CAD build for the part. Positions are in the model's coordinates, mm. Face numbers are marked on the shaded views. A direction names the side the tool comes from. Give positions to 0.01 mm unless a question says otherwise; leave off trailing zeros. Loops run counter-clockwise (first coordinate to the right, second up) from the corner with the lowest first, then second, coordinate; pieces in that order, holes last. Notation, with made-up numbers: M 53,-18 L 92,-18 A22 ccw 92,12 Z; hole C 14.5,-35.75 d3. An arc over 180 degrees is marked long. One line per question, with ' | ' between items.
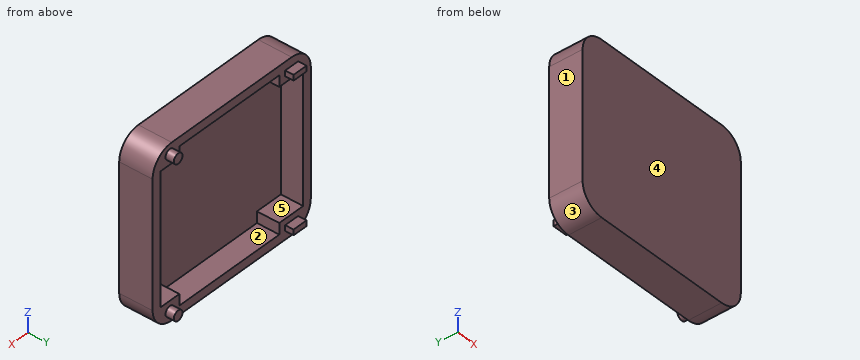
```python
from build123d import *

# Parameters (mm, degrees)
SKETCH1_W           = 84.074
SKETCH1_H           = 77.724
BOSS_EXTRUDE1_DEPTH = 5.08
SKETCH2_W           = 84.074
SKETCH2_H           = 77.724
BOSS_EXTRUDE2_DEPTH = 10.16
FILLET1_R           = 10.16
SKETCH3_R           = 2.286
SKETCH3_W           = 6.858
SKETCH3_H           = 2.54
BOSS_EXTRUDE3_DEPTH = 3.81


with BuildPart() as part:
    # Sketch1 → Boss-Extrude1 (new body)
    with BuildSketch(Plane(origin=(0, 0, 0), x_dir=(1, 0, 0), z_dir=(0, 1, 0))):
        Rectangle(SKETCH1_W, SKETCH1_H)
    extrude(amount=BOSS_EXTRUDE1_DEPTH)

    # Sketch2 → Boss-Extrude2 (add)
    with BuildSketch(Plane(origin=(0, 5.08, 0), x_dir=(1, 0, 0), z_dir=(0, 1, 0))):
        Rectangle(SKETCH2_W, SKETCH2_H)
        Polygon((-37.973, -29.718), (-37.973, 29.718), (-25.273, 29.718), (-25.273, 34.798), (27.813, 34.798), (27.813, 29.718), (37.973, 29.718), (37.973, -29.718), (27.813, -29.718), (27.813, -34.798), (-25.273, -34.798), (-25.273, -29.718), align=None, mode=Mode.SUBTRACT)
    extrude(amount=BOSS_EXTRUDE2_DEPTH)

    # Fillet1
    fillet1_edges = [part.edges().sort_by_distance(p)[0] for p in [
        (42.037, 7.62, 38.862),
        (-42.037, 7.62, 38.862),
        (-42.037, 7.62, -38.862),
        (42.037, 7.62, -38.862),
    ]]
    fillet(fillet1_edges, radius=FILLET1_R)

    # Sketch3 → Boss-Extrude3 (add)
    with BuildSketch(Plane(origin=(0, 15.24, 0), x_dir=(1, 0, 0), z_dir=(0, 1, 0))):
        with Locations((32.893, 34.29)):
            Circle(SKETCH3_R)
        with Locations((-31.877, 33.782)):
            Rectangle(SKETCH3_W, SKETCH3_H)
    boss_extrude3 = extrude(amount=BOSS_EXTRUDE3_DEPTH)

    # Mirror1: Boss-Extrude3 across plane
    add(boss_extrude3.mirror(Plane.XY))


solid = part.part
```
Item 1: Saw through at B-B on x = 23. Give the cut face in (y, z), and give its area (3 significant figures).
Conclusion:
outline: M 0,-38.86 L 15.24,-38.86 L 15.24,-34.8 L 5.08,-34.8 L 5.08,34.8 L 15.24,34.8 L 15.24,38.86 L 0,38.86 Z | area: 477 mm²
Item 2: 3-axis set-ups, long thin cutter, end or side, ignore diameter. For the marked faces 1 and 2: which of +Z, -Z, +X, -X, +Y, -Y reach the whole face in a straight line?
Conclusion:
face 1: +Z, -Z, -X, +Y, -Y | face 2: +Y
Item 3: Drop flat-ended pins along their axis: P1, Ø2.5, axis at y = 8, z = 31.5, coming from the -X side; P2, Ø5, axis at x = -10, z = 0, coming from the -Y side; P3, Ø1.3, axis at y = 16.5, z = -33.5, coming from the -X side; P4, Ø10, axis at x = -3.5, z = -24.5, coming from the +Y side. Give the stop position or say it passes through.
Conclusion:
P1: x = -41.92 | P2: y = 0 | P3: x = -35.31 | P4: y = 5.08
Item 4: Mould opens along Z. For the marked faces 3, 4 and 5 say: pulls with the +Z half, pulls with the -Z half, needs draft (parallel to the pull), parting line crosses it, or undercut.
Conclusion:
face 3: pulls with the -Z half | face 4: needs draft | face 5: undercut
Item 5: Saw through at D-D on y = 8. Give the cut face in (x, z), and give its area (3 significant figures).
Conclusion:
outline: M -42.04,-28.7 A10.16 ccw -31.88,-38.86 L 31.88,-38.86 A10.16 ccw 42.04,-28.7 L 42.04,28.7 A10.16 ccw 31.88,38.86 L -31.88,38.86 A10.16 ccw -42.04,28.7 Z; hole M -37.97,-29.72 L -25.27,-29.72 L -25.27,-34.8 L 27.81,-34.8 L 27.81,-29.72 L 37.97,-29.72 L 37.97,29.72 L 27.81,29.72 L 27.81,34.8 L -25.27,34.8 L -25.27,29.72 L -37.97,29.72 Z | area: 1,390 mm²
Item 6: Saw through at C-C on z = 24. Give the cut face in (x, y), and give its area (3 significant figures).
Conclusion:
outline: M -42.04,0 L 42.04,0 L 42.04,15.24 L 37.97,15.24 L 37.97,5.08 L -37.97,5.08 L -37.97,15.24 L -42.04,15.24 Z | area: 510 mm²
Item 7: Drill centre lines: line 1 along Z through (x, y) = (19, 6.75); line 2 along X through (y, z) = (6.5, -16); line 3 along Z through (x, y) = (31, 14). Where is each one in solid material? Low to high. Write a range as [from, to].
Conclusion:
line 1: [-38.86, -34.8], [34.8, 38.86] | line 2: [-42.04, -37.97], [37.97, 42.04] | line 3: [-38.86, -29.72], [29.72, 38.86]
Item 8: Saw through at A-A on y = 17. Give the cut face in (x, z).
Conclusion:
outline: M -35.31,-35.05 L -28.45,-35.05 L -28.45,-32.51 L -35.31,-32.51 Z; M -35.31,32.51 L -28.45,32.51 L -28.45,35.05 L -35.31,35.05 Z; C 32.89,-34.29 d4.57; C 32.89,34.29 d4.57
